Read the model definition and answer for the solid it produces. Units are mm, in the model's axes. A direction names the side the tool comes from. Coordinates: 2 decimals unless noted, no trailing zeros. Loops run counter-clockwise (first coordinate to the right, second up) from the corner with the lowest first, then second, coordinate; pieces in that order, holes last. Notation, with made-up numbers: (67, 65.5) -> (117, 65.5) arc R29 ccw to (117, 95.5) -> close; hole circle Ø1 at (21.25, 81). An arc over 180 degrees is marked (long way). Answer as a JSON object with one key per item and string values. Group by question number.
1) Flat-ended cylindrical pins translate along their axes: P1, Ø5, axis at y = -3.5, z = 18, coming from the +X side; P2, Ø5, axis at x = -31, y = -3, coming from the +Z side. Find the tip coordinate at first contact, or state that the pin passes through.
2) Section D-D, the plane x = 30.5 is taken. Give the vertices of the cut face in (y, z), plus the area to 3 significant figures.
3) Section C-C, the plane y = -5 is taken. Give the vertices of the cut face in (x, z).
4) Consider probe 1 along Z at (x, y) = (10, -5); probe 2 along Z at (x, y) = (-29, -4.75); probe 3 along Z at (x, y) = (-14, -2). Determine where each line is inside the solid, lowest interval first. Write a range as [from, to].
5) Section A-A, the plane z = -19 is taken. Give the vertices of the cut face in (x, y), plus the area to 3 significant figures.
6) Determine the mould class of faces 1 (the face through (1, 0, -5)), 2 (the face through (0.252, -5.521, 22.966)), 3 (the face through (0, -5, 29)) for opening direction Y: released by +Y, released by -Y, zero draft, split by the parting line, or undercut.
7) Which of the six approach directions +Z, -Z, +X, -X, +Y, -Y give full straight-line access (tool end or side, diameter ignored) to faces 4 (the face through (-28, -5, 9)), 5 (the face through (-1, -5, -24)), 6 (the face through (29, -5, 9))?
8) Section B-B, the plane x = -2 is taken. Give the vertices of the cut face in (y, z), plus the area to 3 significant figures.
from build123d import *

# Parameters (mm, degrees)
F1_DEPTH  = 10
F2_R      = 4
F3_DEPTH  = 38
F4_R      = 4
F5_DEPTH  = 70
F8_DEPTH  = 10
F9_R      = 4
F10_DEPTH = 40
F11_R     = 4
F12_DEPTH = 100
F13_DEPTH = 5
F14_SIZE  = 2


with BuildPart() as f1:
    # F0 (on Front) → F1 (new body)
    with BuildSketch(Plane.XZ):
        Polygon((19, 24), (-19, 24), (-19, 9), (-35, 9), (-35, -24), (35, -24), (35, 9), (19, 9), align=None)
    extrude(amount=F1_DEPTH)

    # F2 (on face) → F3 (cut)
    with BuildSketch(Plane.YZ.offset(19)):
        with Locations((-5, 19)):
            Circle(F2_R)
    extrude(amount=-F3_DEPTH, mode=Mode.SUBTRACT)

    # F4 (on face) → F5 (cut)
    with BuildSketch(Plane.YZ.offset(35)):
        with Locations((-5, -19)):
            Circle(F4_R)
    extrude(amount=-F5_DEPTH, mode=Mode.SUBTRACT)


with BuildPart() as f8:
    # F7 (on Front) → F8 (new body)
    with BuildSketch(Plane.XZ):
        Polygon((18, 24), (-18, 24), (-18, 9), (-39, 9), (-39, -24), (39, -24), (39, 9), (18, 9), align=None)
    extrude(amount=F8_DEPTH)

    # F9 (on face) → F10 (cut)
    with BuildSketch(Plane.YZ.offset(18)):
        with Locations((-5, 19)):
            Circle(F9_R)
    extrude(amount=-F10_DEPTH, mode=Mode.SUBTRACT)

    # F11 (on face) → F12 (cut)
    with BuildSketch(Plane.YZ.offset(39)):
        with Locations((-5, -19)):
            Circle(F11_R)
    extrude(amount=-F12_DEPTH, mode=Mode.SUBTRACT)

    # F13 (add): a face of the model
    f13_faces = [f8.faces().sort_by_distance(p)[0] for p in [
        (0, -5, 24),
    ]]
    extrude(f13_faces, amount=F13_DEPTH)

    # F14
    f14_edges = [f8.edges().sort_by_distance(p)[0] for p in [
        (0, -10, 29),
        (0, 0, 29),
    ]]
    chamfer(f14_edges, length=F14_SIZE)


solid = f8.part
Determined:
{
 "1": {"P1": "x = 18", "P2": "z = 9"},
 "2": {"outline": "(-10, -24) -> (0, -24) -> (0, 9) -> (-10, 9) -> close; hole circle Ø8 at (-5, -19)", "area": "280 mm²"},
 "3": {"outline": "(-39, -24) -> (39, -24) -> (39, -23) -> (-39, -23) -> close; (-39, -15) -> (39, -15) -> (39, 9) -> (18, 9) -> (18, 15) -> (-18, 15) -> (-18, 9) -> (-39, 9) -> close; (-18, 23) -> (18, 23) -> (18, 29) -> (-18, 29) -> close"},
 "4": {"probe 1": "[-24, -23], [-15, 15], [23, 29]", "probe 2": "[-24, -22.99], [-15.01, 9]", "probe 3": "[-24, -21.65], [-16.35, 16.35], [21.65, 29]"},
 "5": {"outline": "(-39, -10) -> (39, -10) -> (39, -9) -> (-39, -9) -> close; (-39, -1) -> (39, -1) -> (39, 0) -> (-39, 0) -> close", "area": "156 mm²"},
 "6": {"face 1": "released by +Y", "face 2": "undercut", "face 3": "zero draft"},
 "7": {"face 4": "+Z, -X, +Y, -Y", "face 5": "-Z, +X, -X, +Y, -Y", "face 6": "+Z, +X, +Y, -Y"},
 "8": {"outline": "(-10, -24) -> (0, -24) -> (0, 27) -> (-2, 29) -> (-8, 29) -> (-10, 27) -> close; hole circle Ø8 at (-5, -19); hole circle Ø8 at (-5, 19)", "area": "425 mm²"}
}
